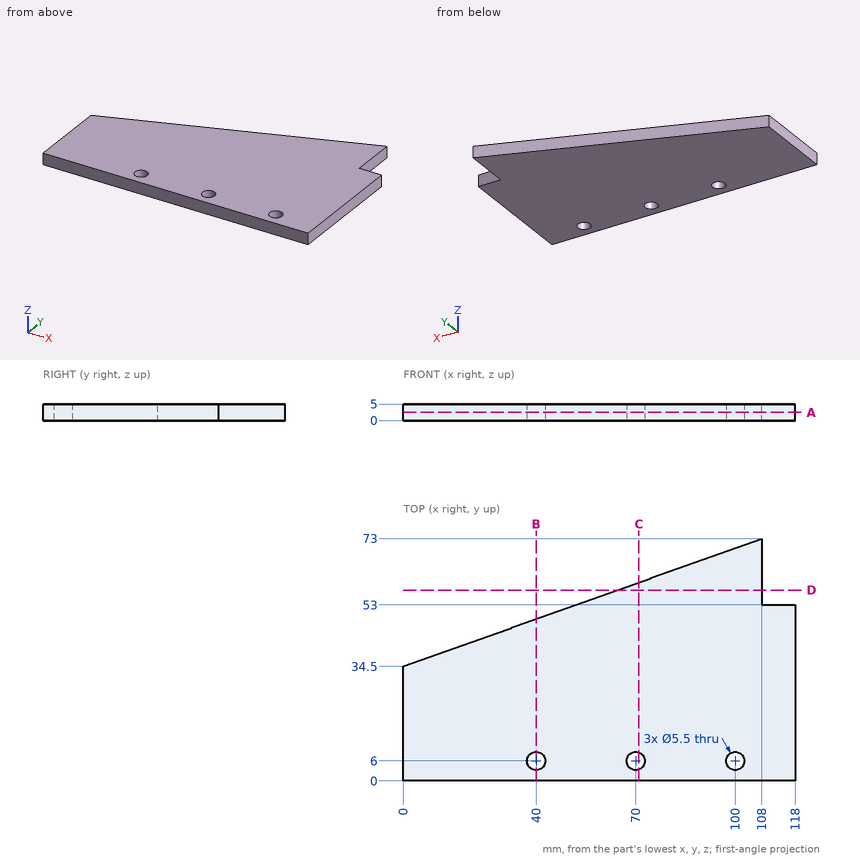
Verification items for this drawing (mm, ordinates from the low corner). Round coordinates to 2 decimals unless told otherwise and drop trailing zeros. Order: outer loops, then holes, each group sorted by start corner. A loop starts at its lowest first (then second) coordinate and runs counter-clockwise, first axis right, second up.
1) Cross-section at B-B, the plane x = 40. Record the cut outline in (y, z), plus the area to 3 significant figures.
Geometry says:
outline: (0, 0) - (3.25, 0) - (3.25, 5) - (0, 5) - close; (8.75, 0) - (48.76, 0) - (48.76, 5) - (8.75, 5) - close
area: 216 mm2
2) Cross-section at D-D, the plane y = 57.5. Record the cut outline in (x, z), plus the area to 3 significant figures.
Geometry says:
outline: (64.52, 0) - (108, 0) - (108, 5) - (64.52, 5) - close
area: 217 mm2
3) Cross-section at A-A, the plane z = 2.5. Record the cut outline in (x, y), plus the area to 3 significant figures.
Geometry says:
outline: (0, 0) - (118, 0) - (118, 53) - (108, 53) - (108, 73) - (0, 34.5) - close; hole circle Ø5.5 at (40, 6); hole circle Ø5.5 at (70, 6); hole circle Ø5.5 at (100, 6)
area: 6,260 mm2
4) Depth check by flat-ended pin: pin 1 (1.5 mm diameter, centred on y = 59.5, z = 1.5, fed in from +X); pin 2 (2.5 mm diameter, centred on x = 112.5, z = 2, fed in from +Y). Enter the tip coordinate at first touch or a pass-through.
Geometry says:
pin 1: stops at x = 108
pin 2: stops at y = 53
5) Material ranges on line 1 (Y direction, x = 40, z = 1.2); line 2 (Y direction, x = 112, z = 0.5); line 3 (Y direction, x = 100, z = 4.05), recorded low to high.
Geometry says:
line 1: y = 0 to 3.25, 8.75 to 48.76
line 2: y = 0 to 53
line 3: y = 0 to 3.25, 8.75 to 70.15
6) Cross-section at C-C, the plane x = 71. Record the cut outline in (y, z), plus the area to 3 significant figures.
Geometry says:
outline: (0, 0) - (3.44, 0) - (3.44, 5) - (0, 5) - close; (8.56, 0) - (59.81, 0) - (59.81, 5) - (8.56, 5) - close
area: 273 mm2
